Input: part model. Units: mm. Frame: model coordinates. Round coordinates to 2 decimals unless told otherwise and drop trailing zeros. Loops run counter-clockwise (first coordinate to the right, second up) from the corner with the lowest first, then second, coordinate; pieces in that order, holes last.
1) Draft query along X for faces 1 (the face through (-6, 18, 0)), 2 (the face through (0, 0, 3)), 3 (the face through (0.54, 16.27, 2.44)). Return one class per face: pulls with the +X half, pulls with the -X half, needs draft (parallel to the pull), parting line crosses it, or undercut.
2) Section C-C, the plane y = 17. Return loops of the section in (x, z), and give its area (3 significant figures).
3) Section D-D, the plane x = 4. Return loops of the section in (y, z).
4) Section A-A, the plane z = 0. Return loops of the section in (x, y), and give its area (3 significant figures).
5) First-contact query: pin 1 (1 mm diameter, centred on y = 17, z = 0, fed in from -X); pin 2 (3.5 mm diameter, centred on x = -8, z = 3, fed in from +Y); pin 3 (5 mm diameter, centred on y = 4.5, z = -2.5, fed in from -X). Flat tips, straight axial feed; report the tip coordinate or a pass-through.
6) Ray query, line 1 along Z through (x, y) = (13.5, 2); line 2 along Z through (x, y) = (0, 19); line 3 along Y through (x, z) = (8, -3.5). Return the intervals inside material, ascending.
from build123d import *

# Parameters (mm, degrees)
SKETCH_1_R          = 6
EXTRUDE_1_DEPTH     = 3
SKETCH_2_R          = 6
EXTRUDE_2_DEPTH     = 30
HOLE_WIZARD_M6_1_D  = 5
SKETCH_6_R          = 3
CUT_EXTRUDE_1_DEPTH = 10


with BuildPart() as part:
    # 草图1 → 凸台-拉伸1 (new body)
    with BuildSketch(Plane(origin=(0, 0, 0), x_dir=(1, 0, 0), z_dir=(0, 1, 0))):
        with Locations((-13.5, 0)):
            Circle(SKETCH_1_R)
        with BuildLine():
            Line((13.5, 6), (-13.5, 6))
            ThreePointArc((-13.5, 6), (-9.257359313, 4.242640687), (-7.5, 0))
            ThreePointArc((-7.5, 0), (-9.257359313, -4.242640687), (-13.5, -6))
            Line((-13.5, -6), (13.5, -6))
            ThreePointArc((13.5, -6), (7.5, 0), (13.5, 6))
        make_face()
        with Locations((13.5, 0)):
            Circle(SKETCH_1_R)
    extrude(amount=EXTRUDE_1_DEPTH)

    # 草图2 → 凸台-拉伸2 (add)
    with BuildSketch(Plane(origin=(0, 3, 0), x_dir=(1, 0, 0), z_dir=(0, 1, 0))):
        Circle(SKETCH_2_R)
    extrude(amount=EXTRUDE_2_DEPTH)

    # M6 螺纹孔1 (through all)
    with Locations(Plane(origin=(0, 33, 0), x_dir=(1, 0, 0), z_dir=(0, 1, 0))):
        with Locations((0, 0)):
            Hole(HOLE_WIZARD_M6_1_D / 2)

    # 草图6 → 切除-拉伸1 (cut)
    with BuildSketch(Plane(origin=(0, 3, 0), x_dir=(1, 0, 0), z_dir=(0, 1, 0))):
        with Locations((-13.5, 0)):
            Circle(SKETCH_6_R)
        with Locations((13.5, 0)):
            Circle(SKETCH_6_R)
    extrude(amount=-CUT_EXTRUDE_1_DEPTH, mode=Mode.SUBTRACT)


solid = part.part
Final values:
1. face 1: parting line crosses it
1. face 2: needs draft
1. face 3: undercut
2. outline: circle Ø12 at (0, 0); hole circle Ø5 at (0, 0)
2. area: 93.5 mm2
3. outline: (0, -6) - (3, -6) - (3, -4.47) - (33, -4.47) - (33, 4.47) - (3, 4.47) - (3, 6) - (0, 6) - close
4. outline: (-19.5, 0) - (-16.5, 0) - (-16.5, 3) - (-19.5, 3) - close; (-10.5, 0) - (-2.5, 0) - (-2.5, 33) - (-6, 33) - (-6, 3) - (-10.5, 3) - close; (2.5, 0) - (10.5, 0) - (10.5, 3) - (6, 3) - (6, 33) - (2.5, 33) - close; (16.5, 0) - (19.5, 0) - (19.5, 3) - (16.5, 3) - close
4. area: 276 mm2
5. pin 1: stops at x = -6
5. pin 2: stops at y = 3
5. pin 3: stops at x = -19.48
6. line 1: z = -6 to -3, 3 to 6
6. line 2: z = -6 to -2.5, 2.5 to 6
6. line 3: y = 0 to 3
